Read the model definition and answer for the solid it produces. Units are mm, in the model's axes. Round coordinates to 2 decimals unless told otherwise and drop trailing zeros. Write each loop counter-clockwise with the first axis right and the second up, starting at its lowest first coordinate (ties: lowest second). Pieces come first, ordered by that corner, then holes. Notation, with made-up numbers: (80, 18) - (118, 18) arc R29 ccw to (118, 39) - close; hole circle Ø9 at (0, 80.5). An arc over 180 degrees is marked (long way). One line per item, written item: value. Start each with the question number.
(1) A cutting plane is placed at A-A, the plane x = -6. Determine the outline of the cut face in (y, z).
(2) Find the intervals of material crossed by L1, parallel to X at y = 1.1, z = 9 (1 decimal); L2, parallel to Z at x = 7, y = 2; L3, parallel to Z at x = 12, y = 3.25, in increasing order.
(3) A cutting plane is placed at D-D, the plane z = -43. Determine the outline of the cut face in (x, y), plus the area to 3 significant figures.
(4) A cutting plane is placed at C-C, the plane x = 17. Determine the outline of the cut face in (y, z), plus the area to 3 significant figures.
(5) Flat-ended cylindrical pins translate along their axes: pin 1 Ø2.5 at (x, z) = (25.46, -20.95) entering from -Y; pin 2 Ø1.6 at (y, z) = (3, -59) entering from -X; pin 3 Ø1.5 at (x, y) = (39, 1) entering from +Z; pin 4 Ø1.4 at (x, y) = (-31, 1.5) entering from -Z. Find the tip coordinate at first contact, or state that the pin passes through.
(6) A cutting plane is placed at B-B, the plane z = 8. Determine the outline of the cut face in (x, y) (1 decimal), plus the area to 3 significant figures.
from build123d import *

# Parameters (mm, degrees)
SKETCH1_R           = 7.3025
SKETCH1_R_2         = 3.6195
SKETCH1_R_3         = 1.55575
SKETCH1_W           = 3.1496
SKETCH1_H           = 35.814
SKETCH1_W_2         = 23.622
SKETCH1_H_2         = 3.1496
BOSS_EXTRUDE2_DEPTH = 4.7625
SKETCH1_4_R         = 3.6195
CUT_EXTRUDE1_DEPTH  = 4.7625


with BuildPart() as part:
    # Sketch1 → Boss-Extrude2 (new body)
    # profile 1 of 17: a face of its own
    with BuildSketch(Plane(origin=(0, 0, 0), x_dir=(1, 0, 0), z_dir=(0, 1, 0))):
        with Locations((25.9715, -58.92165)):
            Circle(SKETCH1_R)
    # profile 2 of 17: a face of its own
    with BuildSketch(Plane(origin=(0, 0, 0), x_dir=(1, 0, 0), z_dir=(0, 1, 0))):
        with Locations((25.9715, -58.92165)):
            Circle(SKETCH1_R_2)
    # profile 3 of 17: a face of its own
    with BuildSketch(Plane(origin=(0, 0, 0), x_dir=(1, 0, 0), z_dir=(0, 1, 0))):
        with Locations((-70.4977, 32.16275)):
            Circle(SKETCH1_R)
    # profile 4 of 17: a face of its own
    with BuildSketch(Plane(origin=(0, 0, 0), x_dir=(1, 0, 0), z_dir=(0, 1, 0))):
        with Locations((-70.4977, 32.16275)):
            Circle(SKETCH1_R_2)
    # profile 5 of 17: a face of its own
    with BuildSketch(Plane(origin=(0, 0, 0), x_dir=(1, 0, 0), z_dir=(0, 1, 0))):
        with Locations((-70.4977, -32.16275)):
            Circle(SKETCH1_R)
    # profile 6 of 17: a face of its own
    with BuildSketch(Plane(origin=(0, 0, 0), x_dir=(1, 0, 0), z_dir=(0, 1, 0))):
        with Locations((-70.4977, -32.16275)):
            Circle(SKETCH1_R_2)
    # profile 7 of 17: a face of its own
    with BuildSketch(Plane(origin=(0, 0, 0), x_dir=(1, 0, 0), z_dir=(0, 1, 0))):
        with Locations((70.4977, 32.16275)):
            Circle(SKETCH1_R)
    # profile 8 of 17: a face of its own
    with BuildSketch(Plane(origin=(0, 0, 0), x_dir=(1, 0, 0), z_dir=(0, 1, 0))):
        with Locations((70.4977, 32.16275)):
            Circle(SKETCH1_R_2)
    # profile 9 of 17: a face of its own
    with BuildSketch(Plane(origin=(0, 0, 0), x_dir=(1, 0, 0), z_dir=(0, 1, 0))):
        with Locations((70.4977, -32.16275)):
            Circle(SKETCH1_R)
    # profile 10 of 17: a face of its own
    with BuildSketch(Plane(origin=(0, 0, 0), x_dir=(1, 0, 0), z_dir=(0, 1, 0))):
        with Locations((70.4977, -32.16275)):
            Circle(SKETCH1_R_2)
    # profile 11 of 17: a face of its own
    with BuildSketch(Plane(origin=(0, 0, 0), x_dir=(1, 0, 0), z_dir=(0, 1, 0))):
        with Locations((25.9715, 58.92165)):
            Circle(SKETCH1_R)
    # profile 12 of 17: a face of its own
    with BuildSketch(Plane(origin=(0, 0, 0), x_dir=(1, 0, 0), z_dir=(0, 1, 0))):
        with Locations((25.9715, 58.92165)):
            Circle(SKETCH1_R_2)
    # profile 13 of 17: a face of its own
    with BuildSketch(Plane(origin=(0, 0, 0), x_dir=(1, 0, 0), z_dir=(0, 1, 0))):
        with Locations((-25.9715, 58.92165)):
            Circle(SKETCH1_R)
    # profile 14 of 17: a face of its own
    with BuildSketch(Plane(origin=(0, 0, 0), x_dir=(1, 0, 0), z_dir=(0, 1, 0))):
        with Locations((-25.9715, 58.92165)):
            Circle(SKETCH1_R_2)
    # profile 15 of 17: a face of its own
    with BuildSketch(Plane(origin=(0, 0, 0), x_dir=(1, 0, 0), z_dir=(0, 1, 0))):
        with Locations((-25.9715, -58.92165)):
            Circle(SKETCH1_R)
    # profile 16 of 17: a face of its own
    with BuildSketch(Plane(origin=(0, 0, 0), x_dir=(1, 0, 0), z_dir=(0, 1, 0))):
        with Locations((-25.9715, -58.92165)):
            Circle(SKETCH1_R_2)
    # profile 17 of 17: a face of its own
    with BuildSketch(Plane(origin=(0, 0, 0), x_dir=(1, 0, 0), z_dir=(0, 1, 0))):
        Polygon((-75.3872, 32.16275), (-75.3872, -32.16275), (-73.016314747, -36.353667562), (-28.490114747, -63.112567562), (-25.9715, -63.81115), (25.9715, -63.81115), (28.490114747, -63.112567562), (73.016314747, -36.353667562), (75.3872, -32.16275), (75.3872, 32.16275), (73.016314747, 36.353667562), (28.490114747, 63.112567562), (25.9715, 63.81115), (-25.9715, 63.81115), (-28.490114747, 63.112567562), (-73.016314747, 36.353667562), align=None)
        with Locations(Location((-25.45715, 20.94865, 0), (0, 0, 90))):
            Circle(SKETCH1_R_3, mode=Mode.SUBTRACT)
        with Locations(Location((25.45715, 20.94865, 0), (0, 0, 90))):
            Circle(SKETCH1_R_3, mode=Mode.SUBTRACT)
        with Locations(Location((25.45715, -20.94865, 0), (0, 0, 90))):
            Circle(SKETCH1_R_3, mode=Mode.SUBTRACT)
        with Locations(Location((-25.45715, -20.94865, 0), (0, 0, 90))):
            Circle(SKETCH1_R_3, mode=Mode.SUBTRACT)
        Polygon((-40.005, 17.907), (-40.005, -17.907), (-22.4155, -17.907), (-22.4155, -25.019), (22.4155, -25.019), (22.4155, -17.907), (40.005, -17.907), (40.005, 17.907), (22.4155, 17.907), (22.4155, 25.019), (-22.4155, 25.019), (-22.4155, 17.907), align=None, mode=Mode.SUBTRACT)
        with Locations((-70.4977, 0)):
            Rectangle(SKETCH1_W, SKETCH1_H, mode=Mode.SUBTRACT)
        with Locations((70.4977, 0)):
            Rectangle(SKETCH1_W, SKETCH1_H, mode=Mode.SUBTRACT)
        with Locations((0, -58.92165)):
            Rectangle(SKETCH1_W_2, SKETCH1_H_2, mode=Mode.SUBTRACT)
        with Locations((0, 58.92165)):
            Rectangle(SKETCH1_W_2, SKETCH1_H_2, mode=Mode.SUBTRACT)
    extrude(amount=BOSS_EXTRUDE2_DEPTH)

    # Sketch1_4 → Cut-Extrude1 (cut, symmetric)
    with BuildSketch(Plane(origin=(0, 0, 0), x_dir=(1, 0, 0), z_dir=(0, 1, 0))):
        with Locations(Location((25.9715, -58.92165, 0), (0, 0, 270))):
            Circle(SKETCH1_4_R)
        with Locations(Location((-70.4977, 32.16275, 0), (0, 0, 270))):
            Circle(SKETCH1_4_R)
        with Locations(Location((-70.4977, -32.16275, 0), (0, 0, 270))):
            Circle(SKETCH1_4_R)
        with Locations(Location((70.4977, 32.16275, 0), (0, 0, 270))):
            Circle(SKETCH1_4_R)
        with Locations(Location((70.4977, -32.16275, 0), (0, 0, 270))):
            Circle(SKETCH1_4_R)
        with Locations(Location((25.9715, 58.92165, 0), (0, 0, 270))):
            Circle(SKETCH1_4_R)
        with Locations(Location((-25.9715, 58.92165, 0), (0, 0, 270))):
            Circle(SKETCH1_4_R)
        with Locations(Location((-25.9715, -58.92165, 0), (0, 0, 270))):
            Circle(SKETCH1_4_R)
    extrude(amount=CUT_EXTRUDE1_DEPTH, both=True, mode=Mode.SUBTRACT)


solid = part.part
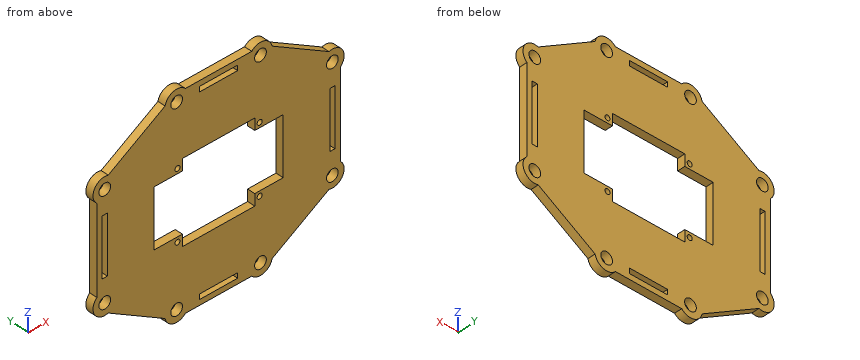
Here are the results:
1. outline: (0, -63.81) - (4.76, -63.81) - (4.76, -60.5) - (0, -60.5) - close; (0, -57.35) - (4.76, -57.35) - (4.76, -25.02) - (0, -25.02) - close; (0, 25.02) - (4.76, 25.02) - (4.76, 57.35) - (0, 57.35) - close; (0, 60.5) - (4.76, 60.5) - (4.76, 63.81) - (0, 63.81) - close
2. L1: -75.4 to -72.1, -68.9 to -40, 40 to 68.9, 72.1 to 75.4
2. L2: -63.81 to -60.5, -57.35 to -25.02, 25.02 to 57.35, 60.5 to 63.81
2. L3: -63.81 to -25.02, 25.02 to 63.81
3. outline: (-61.96, 0) - (61.96, 0) - (61.96, 4.76) - (-61.96, 4.76) - close
3. area: 590 mm²
4. outline: (0, -63.81) - (4.76, -63.81) - (4.76, -25.02) - (0, -25.02) - close; (0, 25.02) - (4.76, 25.02) - (4.76, 63.81) - (0, 63.81) - close
4. area: 369 mm²
5. pin 1: through
5. pin 2: x = -36.66
5. pin 3: z = 57.25
5. pin 4: z = -64.8
6. outline: (-75.4, 0) - (-72.1, 0) - (-72.1, 4.8) - (-75.4, 4.8) - close; (-68.9, 0) - (-40, 0) - (-40, 4.8) - (-68.9, 4.8) - close; (40, 0) - (68.9, 0) - (68.9, 4.8) - (40, 4.8) - close; (72.1, 0) - (75.4, 0) - (75.4, 4.8) - (72.1, 4.8) - close
6. area: 307 mm²
